Drawing for the job (mm, zero at the part's lowest x, y, z). A direction names the side the tool comes from. Give positions to 0.01 mm unless a question says otherwise; leave off trailing zeros. Order: outer loops, then holes, each group sorted by start corner. A loop starts at its lowest first (then second) coordinate and runs counter-clockwise, first axis right, second up. Notation, with made-up numbers: (27, -25.75) -> (53, -25.75) arc R7 cw to (53, -13.75) -> close; hole circle Ø5 at (31.25, -34.5). An arc over 180 degrees is marked (long way). One line per item, written item: value. Start each with the question number.
(1) Saw through at C-C on x = 21.5. Give the cut face in (y, z).
(2) Saw through at B-B on z = 68. Give the cut face in (x, y) (1 decimal).
(3) Probe line 1 (Y direction, x = 17.8, z = 54.75); line 2 (Z direction, x = 25.5, y = 15); line 3 (Y direction, x = 17, z = 56) (1 decimal). List the from-to ranges inside material, lowest first.
(4) Saw through at D-D on z = 9. Give the cut face in (x, y).
(5) Which spindle directions (+Z, -Z, +X, -X, +Y, -Y) get a long thin tool onto all of the face, cutting with end or side? Do the marked faces 1 and 2. Say none if no direction does.
(6) Pin check, flat tips, straight feed: pin 1 (6 mm diameter, centred on y = 7.5, z = 29.5, fed in from -X); pin 2 (10 mm diameter, centred on x = 22.5, y = 10.5, fed in from +Z); pin 3 (4 mm diameter, centred on y = 30, z = 59, fed in from -X). Stop position of each tip, or through.
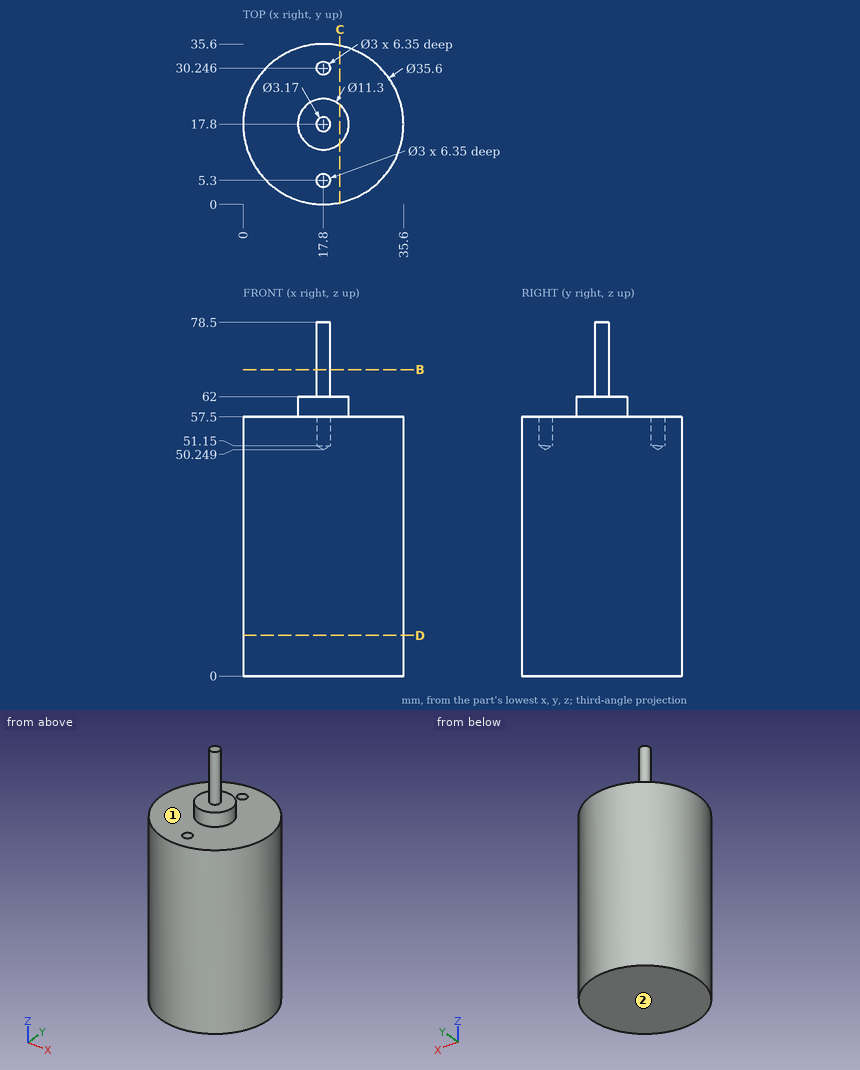
Results below:
1. outline: (0.39, 0) -> (35.21, 0) -> (35.21, 57.5) -> (22.07, 57.5) -> (22.07, 62) -> (13.53, 62) -> (13.53, 57.5) -> (0.39, 57.5) -> close
2. outline: circle Ø3.2 at (17.8, 17.8)
3. line 1: y = 0 to 3.8, 6.8 to 28.75, 31.75 to 35.6
3. line 2: z = 0 to 57.5
3. line 3: y = 0 to 4, 6.6 to 29, 31.5 to 35.6
4. outline: circle Ø35.6 at (17.8, 17.8)
5. face 1: +Z
5. face 2: -Z, +X, -X, +Y, -Y
6. pin 1: stops at x = 1.57
6. pin 2: stops at z = 62
6. pin 3: stops at x = 3.71
